```python
from build123d import *

# Parameters (mm, degrees)
POCKET001_DEPTH       = 197.910551
POLARPATTERN001_COUNT = 4
HOLE001_D             = 3.4
HOLE001_CBORE_D       = 6.1
HOLE001_CBORE_DEPTH   = 3.6


with BuildPart() as part:
    # Sketch019 → Revolution001 (revolve)
    with BuildSketch(Plane.XZ):
        with BuildLine():
            Line((31.5, 9), (31.5, 0))
            Line((31.5, 0), (34.5, 0))
            Line((34.5, 0), (34.5, -0.4))
            Line((34.5, -0.4), (33.3, -1.6))
            Line((33.3, -1.6), (0, -1.6))
            Line((0, -1.6), (0, 9))
            Line((0, 9), (4, 9))
            Line((4, 9), (4, 1))
            ThreePointArc((4, 1), (4.292893, 0.292893), (5, 0))
            Line((5, 0), (29.9, 0))
            Line((29.9, 0), (29.9, 9))
            Line((29.9, 9), (31.5, 9))
        make_face()
    revolve(axis=Axis((0, 0, 0), (0, 0, 1)))

    # Sketch020 → Pocket001 (cut, through all)
    with BuildSketch(Plane.XY):
        with BuildLine():
            ThreePointArc((29.757016, 1.6), (21.071782, 21.071782), (1.6, 29.757016))
            Line((1.6, 29.757016), (1.6, 5.574944))
            ThreePointArc((5.574944, 1.6), (4.101219, 4.101219), (1.6, 5.574944))
            Line((5.574944, 1.6), (29.757016, 1.6))
        make_face()
    pocket001 = extrude(amount=-POCKET001_DEPTH, mode=Mode.SUBTRACT)

    # PolarPattern001: Pocket001 ×4 about axis
    polarpattern001_axis = Axis((0, 0, 0), (0, 0, 1))
    for i in range(1, POLARPATTERN001_COUNT):
        add(pocket001.rotate(polarpattern001_axis, i * 360 / POLARPATTERN001_COUNT), mode=Mode.SUBTRACT)

    # Hole001 (through all)
    with Locations(Plane(origin=(0, 0, -1.6), x_dir=(1, 0, 0), z_dir=(0, 0, -1))):
        with Locations((0, 0)):
            CounterBoreHole(HOLE001_D / 2, HOLE001_CBORE_D / 2, HOLE001_CBORE_DEPTH)


with BuildPart() as part_1:
    # Body001 placement: moved
    add(part.part.moved(Location((0, 0, -19))))


solid = part_1.part
```
Geometry check sheet. Reference: the model listing, model coordinates, mm. A direction names the side the tool comes from. Round coordinates to 2 decimals unless told otherwise and drop trailing zeros. Loops run counter-clockwise (first coordinate to the right, second up) from the corner with the lowest first, then second, coordinate; pieces in that order, holes last. Notation, with made-up numbers: M 28,-16 L 38,-16 A33 ccw 38,14 Z; hole C 81.5,12 d7. An arc over 180 degrees is marked long. Return JSON: item names as keys, results as strings. Group by question number.
(1) Scan lines: line 1 along Y through (x, z) = (0, -15); line 2 along Y through (x, z) = (0, -18.1); line 3 along X through (y, z) = (-1, -15.5). Record each from-to range of solid material in increasing order. Write a range as [from, to].
(2) Mould release check, pull along Y, two halves, no side actions. Record for faces 1 (the face through (-4.101, 31.232, -14.563)), 2 (the face through (-15, -28, -19)), 3 (the face through (18, -1.6, -20)): pulls with the +Y half, pulls with the -Y half, needs draft (parallel to the pull), parting line crosses it, or undercut.
(3) Go/stop test with flat-tipped pins: pin 1 (0.8 mm diameter, centred on y = -12.5, z = -20, fed in from -X); pin 2 (0.5 mm diameter, centred on x = -18, z = -19.5, fed in from +Y); pin 3 (0.5 mm diameter, centred on x = 17.5, z = -19.5, fed in from -Y); pin 4 (2 mm diameter, centred on x = 0, y = 0, fed in from -Z). Record where each tip stops, or that it passes through.
(4) Section check D-D, the plane x = -14. Give the number of separate pieces and of enclosed holes in the cut face, and give its area (3 significant figures).
(5) Set-up check for faces 4 (the face through (1.31, 1.31, -17)), 5 (the face through (0, -7, -20.6)), 6 (the face through (13.797, -26.526, -14.437)), 7 (the face through (-18, 1.6, -20)): record each of +Z, -Z, +X, -X, +Y, -Y from which the full face is reachable in a straight line by a thin tool's end or side.
(6) Section check A-A, the plane x = 0. Enter the section's corners in (y, z).
(7) Section check C-C, the plane z = -16. Enter the section's corners in (x, y), and give its area (3 significant figures).
Data:
{
 "1": {"line 1": "[-31.5, -29.9], [-4, -1.7], [1.7, 4], [29.9, 31.5]", "line 2": "[-31.5, -29.9], [-4.01, -3.05], [3.05, 4.01], [29.9, 31.5]", "line 3": "[-31.48, -29.88], [-3.87, -1.37], [1.37, 3.87], [29.88, 31.48]"},
 "2": {"face 1": "parting line crosses it", "face 2": "needs draft", "face 3": "undercut"},
 "3": {"pin 1": "x = -31.97", "pin 2": "y = 29.57", "pin 3": "y = -29.87", "pin 4": "through"},
 "4": {"separate pieces": "3", "enclosed holes": "0", "area": "52.6 mm²"},
 "5": {"face 4": "-Z", "face 5": "-Z, +X, -X, +Y, -Y", "face 6": "+Z", "face 7": "+Z, -Z"},
 "6": {"outline": "M -34.5,-19.4 L -33.3,-20.6 L -3.05,-20.6 L -3.05,-17 L -1.7,-17 L -1.7,-10 L -4,-10 L -4,-18 A1 cw -5,-19 L -29.9,-19 L -29.9,-10 L -31.5,-10 L -31.5,-19 L -34.5,-19 Z; M 1.7,-17 L 3.05,-17 L 3.05,-20.6 L 33.3,-20.6 L 34.5,-19.4 L 34.5,-19 L 31.5,-19 L 31.5,-10 L 29.9,-10 L 29.9,-19 L 5,-19 A1 cw 4,-18 L 4,-10 L 1.7,-10 Z"},
 "7": {"outline": "C 0,0 d63; C 0,0 d8; hole C 0,0 d59.8; hole C 0,0 d3.4", "area": "350 mm²"}
}
